from build123d import *

# Parameters (mm, degrees)
BOSS_EXTRUDE1_DEPTH     = 7.5
LPATTERN1_COUNT         = 8
LPATTERN1_PITCH         = 10
LPATTERN1_COL_COUNT     = 8
LPATTERN1_COL_PITCH     = 10
SHELL2_T                = -2
CUT_EXTRUDE2_DEPTH      = 15
CUT_EXTRUDE2_DEPTH_BACK = 80.411900871
SKETCH3_W               = 1
SKETCH3_H               = 7
SKETCH4_W               = 11
SKETCH4_H               = 3
BOSS_EXTRUDE2_DEPTH     = 2
SKETCH5_W               = 11
SKETCH5_H               = 4
BOSS_EXTRUDE3_DEPTH     = 2
SKETCH6_W               = 148
SKETCH6_H               = 1
BOSS_EXTRUDE4_DEPTH     = 7.5
SKETCH8_W               = 8
SKETCH8_H               = 15
BOSS_EXTRUDE5_DEPTH     = 1
LPATTERN2_COUNT         = 15
LPATTERN2_PITCH         = 10
SKETCH10_W              = 8
SKETCH10_H              = 15
CUT_EXTRUDE4_DEPTH      = 21
SKETCH11_W              = 15
SKETCH11_H              = 2
BOSS_EXTRUDE6_DEPTH     = 8


# Read off the part's stored shape, not the designer's step: Split1
with BuildPart() as part:
    # Sketch1 → Boss-Extrude1 (new, symmetric)
    with BuildSketch(Plane.XY):
        Polygon((0, 0), (-5, 0), (-5, 7), (-4, 7), (-4, 25), (4, 25), (4, 7), (5, 7), (5, 0), align=None)
    boss_extrude1 = extrude(amount=BOSS_EXTRUDE1_DEPTH, both=True)

    # LPattern1: Boss-Extrude1 ×8
    with Locations(*[(-i * LPATTERN1_PITCH, 0, 0) for i in range(1, LPATTERN1_COUNT)]):
        add(boss_extrude1)


with BuildPart() as lpattern1_col_1:
    # LPattern1 col: pattern copy
    add(boss_extrude1.moved(Location(Vector(1, 0, 0) * (1 * LPATTERN1_COL_PITCH))))


with BuildPart() as lpattern1_col_2:
    # LPattern1 col: pattern copy
    add(boss_extrude1.moved(Location(Vector(1, 0, 0) * (2 * LPATTERN1_COL_PITCH))))


with BuildPart() as lpattern1_col_3:
    # LPattern1 col: pattern copy
    add(boss_extrude1.moved(Location(Vector(1, 0, 0) * (3 * LPATTERN1_COL_PITCH))))


with BuildPart() as lpattern1_col_4:
    # LPattern1 col: pattern copy
    add(boss_extrude1.moved(Location(Vector(1, 0, 0) * (4 * LPATTERN1_COL_PITCH))))


with BuildPart() as lpattern1_col_5:
    # LPattern1 col: pattern copy
    add(boss_extrude1.moved(Location(Vector(1, 0, 0) * (5 * LPATTERN1_COL_PITCH))))


with BuildPart() as lpattern1_col_6:
    # LPattern1 col: pattern copy
    add(boss_extrude1.moved(Location(Vector(1, 0, 0) * (6 * LPATTERN1_COL_PITCH))))


with BuildPart() as lpattern1_col_7:
    # LPattern1 col: pattern copy
    add(boss_extrude1.moved(Location(Vector(1, 0, 0) * (7 * LPATTERN1_COL_PITCH))))


with BuildPart() as part_1:
    add(part.part)

    # LPattern1 col united with what the copie: union LPattern1 col_1, LPattern1 col_2, LPattern1 col_3, LPattern1 col_4, LPattern1 col_5, LPattern1 col_6, LPattern1 col_7
    add(lpattern1_col_1.part)
    add(lpattern1_col_2.part)
    add(lpattern1_col_3.part)
    add(lpattern1_col_4.part)
    add(lpattern1_col_5.part)
    add(lpattern1_col_6.part)
    add(lpattern1_col_7.part)

    # Shell2
    shell2_openings = [part_1.faces().sort_by_distance(p)[0] for p in [
        (75, 3.5, 0),
        (-75, 3.5, 0),
    ]]
    offset(amount=SHELL2_T, openings=shell2_openings, kind=Kind.INTERSECTION)

    # Sketch3 → Cut-Extrude2 (cut, two sides: drawn at the far end of the back side and taken through both)
    with BuildSketch(Plane.XY.offset(-CUT_EXTRUDE2_DEPTH_BACK)):
        with Locations((-74.5, 3.5)):
            Rectangle(SKETCH3_W, SKETCH3_H)
        with Locations((74.5, 3.5)):
            Rectangle(SKETCH3_W, SKETCH3_H)
    extrude(amount=CUT_EXTRUDE2_DEPTH + CUT_EXTRUDE2_DEPTH_BACK, mode=Mode.SUBTRACT)

    # Sketch4 → Boss-Extrude2 (add)
    with BuildSketch(Plane.ZY.offset(74)):
        with Locations((0, 3.5)):
            Rectangle(SKETCH4_W, SKETCH4_H)
    extrude(amount=-BOSS_EXTRUDE2_DEPTH)

    # Sketch5 → Boss-Extrude3 (add)
    with BuildSketch(Plane(origin=(74, 0, 0), x_dir=(0, 0, -1), z_dir=(1, 0, 0))):
        with Locations((0, 3)):
            Rectangle(SKETCH5_W, SKETCH5_H)
    extrude(amount=-BOSS_EXTRUDE3_DEPTH)

    # Sketch6 → Boss-Extrude4 (add, symmetric)
    with BuildSketch(Plane.XY):
        with Locations((0, -0.5)):
            Rectangle(SKETCH6_W, SKETCH6_H)
    extrude(amount=BOSS_EXTRUDE4_DEPTH, both=True)

    # Sketch8 → Boss-Extrude5 (add)
    with BuildSketch(Plane(origin=(0, 25, 0), x_dir=(1, 0, 0), z_dir=(0, 1, 0))):
        with Locations((-70, 0)):
            Rectangle(SKETCH8_W, SKETCH8_H)
    boss_extrude5 = extrude(amount=BOSS_EXTRUDE5_DEPTH)

    # LPattern2: Boss-Extrude5 ×15
    with Locations(*[(i * LPATTERN2_PITCH, 0, 0) for i in range(1, LPATTERN2_COUNT)]):
        add(boss_extrude5)


with BuildPart() as body_2:
    # Split1: the piece on the far side of the plane
    add(part_1.part)
    split(bisect_by=Plane(origin=(0, 2, 0), x_dir=(1, 0, 0), z_dir=(0, 1, 0)), keep=Keep.BOTTOM)


with BuildPart() as part_2:
    add(part_1.part)

    # Split1
    split(bisect_by=Plane(origin=(0, 2, 0), x_dir=(1, 0, 0), z_dir=(0, 1, 0)), keep=Keep.TOP)

    # Sketch10 → Cut-Extrude4 (cut)
    with BuildSketch(Plane(origin=(0, 26, 0), x_dir=(1, 0, 0), z_dir=(0, 1, 0))):
        Rectangle(SKETCH10_W, SKETCH10_H)
    extrude(amount=-CUT_EXTRUDE4_DEPTH, mode=Mode.SUBTRACT)

    # Sketch11 → Boss-Extrude6 (add)
    with BuildSketch(Plane(origin=(-4, 0, 0), x_dir=(0, 0, -1), z_dir=(1, 0, 0))):
        with Locations((0, 6)):
            Rectangle(SKETCH11_W, SKETCH11_H)
    extrude(amount=BOSS_EXTRUDE6_DEPTH)


with BuildPart() as body_2_1:
    add(body_2.part)

    # Combine1: union part
    add(part_2.part)


solid = body_2_1.part
Model file for the job. Use its own axes, mm. A direction names the side the tool comes from. Give positions to 0.01 mm unless a question says otherwise; leave off trailing zeros. Write item = value, one per line.
(1) Slice it at A-A, the plane y = 10.5. Give the number of separate pieces and of enclosed holes in the cut face, then the cut area to 3 significant figures.
Determined:
separate_pieces = 14
enclosed_holes = 14
area = 1,060 mm2
(2) Probe line 1 along Y through (x, z) = (5.5, 3); line 2 along Z through (x, y) = (-51, 17.75); line 3 along X through (y, z) = (3, 4.25). List the from-to ranges inside material, lowest first.
Determined:
line_1 = -1 to 2, 5 to 7
line_2 = -7.5 to -5.5, 5.5 to 7.5
line_3 = -74 to -72, 72 to 74
(3) Mould opens along Y. For faces 4 (the face through (-16, 17, 0)), 5 (the face through (-38, 14, 0)), 6 (the face through (60, 23, 0)), 7 (the face through (50, 26, 0)) say: released by +Y, released by -Y, zero draft, split by the parting line, or undercut.
Determined:
face_4 = zero draft
face_5 = undercut
face_6 = undercut
face_7 = released by +Y
(4) Tool access for faces 1 (the face through (-44, 16, 0)), 2 (the face through (-10, 26, 0)), 3 (the face through (45, 5, 0)): list every direction of +Z, -Z, +X, -X, +Y, -Y with a clear straight run to the whole face (end or side of a thin tool).
Determined:
face_1 = +Z, -Z, +Y
face_2 = +Z, -Z, +X, -X, +Y
face_3 = none
(5) Flat gauge pin, fed straight in: P1, Ø1.6, axis at x = 15, z = 2.5, coming from the +Y side. Where does the tip first touch, or does it go through?
Determined:
P1 = 7
